Part print with two shaded views. Sizes in mm from the minimum x, y, z corner. A direction names the side the tool comes from. Coordinates: 2 decimals unless noted, no trailing zeros. Loops run counter-clockwise (first coordinate to the right, second up) from the corner with the lowest first, then second, coordinate; pieces in that order, holes last. Notation, with made-up numbers: (52.25, -17) - (109.25, -17) arc R30 cw to (109.25, 18) - close; hole circle Ø7 at (-39, -0.75). An arc over 180 degrees is marked (long way). Answer as CSV lines item,"result".
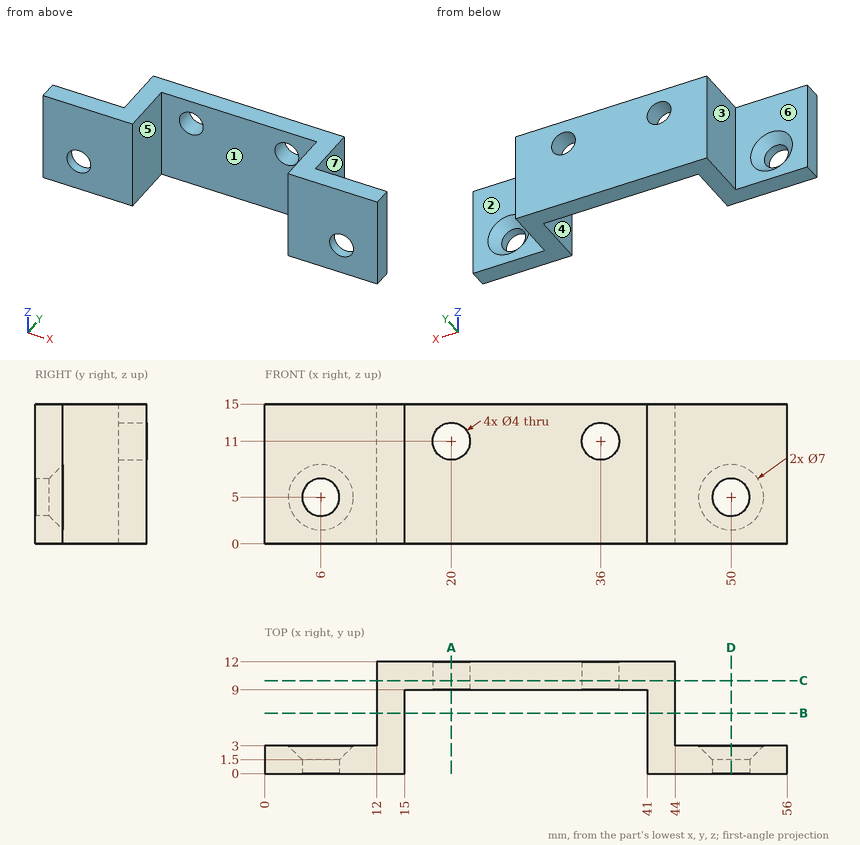
Q1. Which spindle directions (+Z, -Z, +X, -X, +Y, -Y) get a long thin tool onto all of the face, cutting with end or side? Do the marked faces 1, 2 and 3. Say none if no direction does.
Results:
face 1,"+Z, -Z, -Y"
face 2,"+Z, -Z, +X, +Y"
face 3,"+Z, -Z, -X, +Y"
Q2. Saw through at C-C (y = 10). Give the cut face in (x, z).
Results:
outline,"(12, 0) - (44, 0) - (44, 15) - (12, 15) - close; hole circle Ø4 at (20, 11); hole circle Ø4 at (36, 11)"
Q3. Saw through at D-D (x = 50). Give the cut face in (y, z).
Results:
outline,"(0, 0) - (3, 0) - (3, 1.5) - (1.5, 3) - (0, 3) - close; (0, 7) - (1.5, 7) - (3, 8.5) - (3, 15) - (0, 15) - close"
Q4. Two-plate mould, pull along X, no slides. Class the marked faces 4, 5, 6 and 7: released by +X, released by -X, zero draft, split by the parting line, or undercut.
Results:
face 4,"undercut"
face 5,"undercut"
face 6,"zero draft"
face 7,"released by +X"
Q5. Saw through at B-B (y = 6.5). Give the cut face in (x, z).
Results:
outline,"(12, 0) - (15, 0) - (15, 15) - (12, 15) - close; (41, 0) - (44, 0) - (44, 15) - (41, 15) - close"
Q6. Wall check: L1, parallel to X at y = 1.1, z = 5; L2, parallel to X at y = 6, z = 3.75; L3, parallel to Z at x = 20, y = 11.15. Give the ranges that are in metal, low to high.
Results:
L1,"x = 0 to 4, 8 to 15, 41 to 48, 52 to 56"
L2,"x = 12 to 15, 41 to 44"
L3,"z = 0 to 9, 13 to 15"
Q7. Flat gauge pins, fed straight in: pin 1 (4.5 mm diameter, centred on x = 28.5, z = 11, fed in from -Y); pin 2 (1.5 mm diameter, centred on y = 7, z = 9, fed in from -X); pin 3 (2.5 mm diameter, centred on x = 6, z = 5, fed in from +Y). Where does each tip first touch, or does it go through?
Results:
pin 1,"stops at y = 9"
pin 2,"stops at x = 12"
pin 3,"passes through"
Q8. Saw through at A-A (x = 20). Give the cut face in (y, z), then the cut area to 3 significant figures.
Results:
outline,"(9, 0) - (12, 0) - (12, 9) - (9, 9) - close; (9, 13) - (12, 13) - (12, 15) - (9, 15) - close"
area,"33.0 mm^2"
